For this review, take the finished solid that the model builds, in its own axes (mm). A direction names the side the tool comes from. Give positions to 0.01 mm unless a question says otherwise; leave off trailing zeros. Order: outer loops, then holes, each group sorted by start corner. A loop starts at its lowest first (then second) coordinate and runs counter-clockwise, first axis right, second up. Notation, with made-up numbers: (3.5, -32) -> (42.5, -32) arc R17 ccw to (42.5, -15) -> close; hole circle Ø10 at (-28.5, -34.75). An arc over 180 degrees is marked (long way). One line per item, written item: value. Start each with the question number.
from build123d import *

# Parameters (mm, degrees)
F0_W     = 1000
F0_H     = 250
F1_DEPTH = 1.5
F3_D     = 11
F3_DEPTH = 18
F3_TIP   = 3.3047334047
F4_R     = 5.5
F5_DEPTH = 3.001
F6_R     = 50


with BuildPart() as f1:
    # F0 (on Front) → F1 (new body, symmetric)
    with BuildSketch(Plane.XZ):
        Rectangle(F0_W, F0_H)
    extrude(amount=F1_DEPTH, both=True)

    # F3
    with Locations(Plane.XZ.offset(1.5)):
        with Locations((-475, 56.2), (-475, -100), (-425, -105.7), (-425, 45.1), (-75, -28), (75, -28), (0, -105.7), (0, 45.1), (245, 45.1), (245, -105.7)):
            Hole(F3_D / 2, depth=F3_DEPTH)
            with Locations((0, 0, -(F3_DEPTH + F3_TIP / 2))):  # 118° drill point
                Cone(0, F3_D / 2, F3_TIP, mode=Mode.SUBTRACT)

    # F4 (on face) → F5 (cut, through all)
    with BuildSketch(Plane(origin=(0, 1.5, 0), x_dir=(-1, 0, 0), z_dir=(0, 1, 0))):
        with Locations((-372.5, -30)):
            Circle(F4_R)
        with Locations((-372.5, 69)):
            Circle(F4_R)
        with BuildLine():
            ThreePointArc((-410, 39.5), (-430, 19.5), (-410, -0.5))
            Line((-410, -0.5), (-335, -0.5))
            ThreePointArc((-335, -0.5), (-315, 19.5), (-335, 39.5))
            Line((-335, 39.5), (-410, 39.5))
        make_face()
    extrude(amount=-F5_DEPTH, mode=Mode.SUBTRACT)

    # F6
    f6_edges = [f1.edges().sort_by_distance(p)[0] for p in [
        (500, 0, 125),
        (500, 0, -125),
    ]]
    fillet(f6_edges, radius=F6_R)


solid = f1.part
Q1. Take a section at A-A (y = 0.4). State how many separate pieces and enclosed holes the cut face has, and give its area (3 significant figures).
Q2. Take a section at B-B (z = 24). State the section outline as (x, y) points, and give its area (3 significant figures).
Q3. For pin 1 Ø17.5 at (x, z) = (-75, -28) entering from +Y; pin 2 Ø9 at (x, z) = (372.5, -30) entering from +Y, all flat-tipped, find the tip position at first contact; note any pin that passes through.
Q4. Mouldability with a two-part tool opening along Z and no side actions: class faces 1 (the cylindrical face through (429.995, 0.021, 19.94)), 2 (the flat face through (-7, -1.5, 2)), 3 (the cylindrical face through (484.964, -0.021, -110.742)) as pulls with the +Z half, pulls with the -Z half, needs draft (parallel to the pull), parting line crosses it, or undercut.
Q5. For faces 4 (the cylindrical face through (484.964, 0.021, 110.742)), 5 (the cylindrical face through (315.005, 0.021, 19.06)), list the 3-axis set-ups (+Z, -Z, +X, -X, +Y, -Y) from which the entire face can be reached by the end or side of a thin tool; tool diameter is ignored.
Q6. For line 1 along Z through (x, y) = (245, -0.6); line 2 along Z through (x, y) = (372.5, -0.7); line 3 along X through (y, z) = (0.85, 49), list the stretches that pass through material, from the lowest coordinate up.
Answers below:
1. separate pieces: 1
1. enclosed holes: 13
1. area: 244,000 mm²
2. outline: (-500, -1.5) -> (315.51, -1.5) -> (315.51, 1.5) -> (-500, 1.5) -> close; (429.49, -1.5) -> (500, -1.5) -> (500, 1.5) -> (429.49, 1.5) -> close
2. area: 2,660 mm²
3. pin 1: stops at y = 1.5
3. pin 2: passes through
4. face 1: undercut
4. face 2: needs draft
4. face 3: pulls with the -Z half
5. face 4: +Z, +X, +Y, -Y
5. face 5: +Y, -Y
6. line 1: z = -125 to -111.2, -100.2 to 39.6, 50.6 to 125
6. line 2: z = -125 to -35.5, -24.5 to -0.5, 39.5 to 63.5, 74.5 to 125
6. line 3: x = -500 to -428.88, -421.12 to -3.88, 3.88 to 241.12, 248.88 to 500
